Autodesk Fusion 360 part; units mm, degrees
sketch "Sketch1" plane through (0, 0, 0) normal (0, 0, 1) x (1, 0, 0)
  line L0 (0, 0) -> (21, 0)
  line L1 (21, 0) -> (21, 2)
  line L2 (21, 2) -> (0, 2)
  line L3 (0, 2) -> (0, 0)
  line L4 (0, 2) -> (2, 2)
  line L5 (2, 2) -> (2, -18)
  line L6 (2, -18) -> (0, -18)
  line L7 (0, -18) -> (0, 2)
  line L8 (21, 2) -> (19, 2)
  line L9 (19, 2) -> (19, -23)
  line L10 (19, -23) -> (21, -23)
  line L11 (21, -23) -> (21, 2)
  line L12 (19, -23) -> (34, -23)
  line L13 (34, -23) -> (34, -25)
  line L14 (34, -25) -> (19, -25)
  line L15 (19, -25) -> (19, -23)
  line L16 (34, -23) -> (32, -23)
  line L17 (32, -23) -> (32, -11)
  line L18 (32, -11) -> (34, -11)
  line L19 (34, -11) -> (34, -23)
  dimension "d1" = 21
  dimension "d2" = 2
  dimension "d3" = 2
  dimension "d4" = 20
  dimension "d5" = 2
  dimension "d6" = 25
  dimension "d7" = 15
  dimension "d8" = 2
  dimension "d9" = 2
  dimension "d10" = 12
extrude "Extrude1" add sketch "Sketch1" along normal blind 10
fillet "Fillet1" radius 4 2 edges at (21, -23, 5) (32, -23, 5)
The listing builds one solid part. Answer for the finished solid, in the listing's coordinates (mm). A direction names the side the tool comes from. Give positions to 0.01 mm unless a question says otherwise; leave off trailing zeros. Write each loop counter-clockwise with the first axis right and the second up, starting at its lowest first coordinate (ties: lowest second). Pieces come first, ordered by that corner, then holes.
Item 1: Flat-ended cylindrical pins translate along their axes: P1, Ø5, axis at y = -17, z = 7.5, coming from the -X side; P2, Ø5, axis at x = 9.5, z = 4.5, coming from the -Y side; P3, Ø5, axis at y = -4, z = 4, coming from the +X side; P4, Ø3.5, axis at x = 26.5, z = 6.5, coming from the +Y side. Find the tip coordinate at first contact, or state that the pin passes through.
Item 2: Which of the six approach directions +Z, -Z, +X, -X, +Y, -Y give full straight-line access (tool end or side, diameter ignored) to faces 1 (the flat face through (1, -18, 5)), 2 (the cylindrical face through (30.797, -21.859, 5.07)), 3 (the flat face through (11, 2, 5)), 4 (the flat face through (2, -9, 5))?
Item 3: Section D-D, the plane x = 30 is taken. Write down the section's boundary in (y, z), plus the area to 3 significant figures.
Item 4: Determine the mould class of faces 5 (the flat face through (10, 0, 5)), 6 (the flat face through (0, -8, 5)), 7 (the flat face through (19, -12, 5)), 8 (the flat face through (33, -11, 5)) for opening direction X: released by +X, released by -X, zero draft, split by the parting line, or undercut.
Item 5: Find the intervals of material crossed by line 1 along X through (y, z) = (-16.5, 1.75); line 2 along X through (y, z) = (-6, 7.25); line 3 along Y through (x, z) = (13, 4), in increasing order.
Item 6: Section C-C, the plane x = 15 is taken. Write down the section's boundary in (y, z), plus the area to 3 significant figures.
Item 7: Section B-B, the plane z = 1.5 is taken. Write down the section's boundary in (x, y), plus the area to 3 significant figures.
Item 8: Section A-A, the plane y = -8.25 is taken. Write down the section's boundary in (x, z), plus the area to 3 significant figures.
Completed:
1. P1: stops at x = 0
1. P2: stops at y = 0
1. P3: stops at x = 21
1. P4: stops at y = -22.99
2. face 1: +Z, -Z, -X, -Y
2. face 2: +Z, -Z, +Y
2. face 3: +Z, -Z, +X, -X, +Y
2. face 4: +Z, -Z, -Y
3. outline: (-25, 0) - (-22.46, 0) - (-22.46, 10) - (-25, 10) - close
3. area: 25.4 mm2
4. face 5: undercut
4. face 6: released by -X
4. face 7: undercut
4. face 8: zero draft
5. line 1: x = 0 to 2, 19 to 21, 32 to 34
5. line 2: x = 0 to 2, 19 to 21
5. line 3: y = 0 to 2
6. outline: (0, 0) - (2, 0) - (2, 10) - (0, 10) - close
6. area: 20.0 mm2
7. outline: (0, -18) - (2, -18) - (2, 0) - (19, 0) - (19, -25) - (34, -25) - (34, -11) - (32, -11) - (32, -19) arc R4 cw to (28, -23) - (25, -23) arc R4 cw to (21, -19) - (21, 2) - (0, 2) - close
7. area: 185 mm2
8. outline: (0, 0) - (2, 0) - (2, 10) - (0, 10) - close; (19, 0) - (21, 0) - (21, 10) - (19, 10) - close
8. area: 40.0 mm2
